The model under review builds one solid part; all positions refer to its coordinate system, in mm. A direction names the side the tool comes from. Round coordinates to 2 decimals unless told otherwise and drop trailing zeros. Order: outer loops, then holes, each group sorted by start corner. A loop starts at its lowest first (then second) coordinate and runs counter-clockwise, first axis right, second up. Notation, with made-up numbers: M 25,-13 L 78,-13 A22 cw 78,-6 Z; hole C 78.25,66.25 d6. An arc over 180 degrees is marked long. Answer as CSV lines item,"result". Start each with the question number.
from build123d import *

# Parameters (mm, degrees)
SKETCH2_W         = 27.0256
SKETCH2_H         = 28.448
MOUNT_BLOCK_DEPTH = 22.2123
MID_HEX_DEPTH     = 20.7645
SKETCH4_R         = 4.233333333
SKETCH4_R_2       = 3.175
SWGLK_M_DEPTH     = 10.287
SKETCH6_R         = 6.35
SKETCH6_R_2       = 3.175
SKETCH7_R         = 2.05105
MOUNT_HOLES_DEPTH = 12.7


with BuildPart() as part:
    # Sketch1 → BASE (revolve)
    with BuildSketch(Plane(origin=(0, 0, 0), x_dir=(0, 0, -1), z_dir=(1, 0, 0)), mode=Mode.PRIVATE) as base_sk:
        Polygon((0, 0), (12.7, 0), (12.7, 22.2123), (14.21765, 22.2123), (14.21765, 42.9768), (9.4234, 42.9768), (9.4234, 51.0667), (26.924, 51.0667), (26.924, 99.1743), (0, 99.1743), align=None)
    revolve(base_sk.sketch.rotate(Axis((0, 0, 0), (0, -1, 0)), 180), axis=Axis((0, 0, 0), (0, -1, 0)))

    # Sketch2 → MOUNT_BLOCK (add)
    with BuildSketch(Plane.XZ):
        Rectangle(SKETCH2_W, SKETCH2_H)
    extrude(amount=-MOUNT_BLOCK_DEPTH)

    # Sketch3 → MID_HEX (add)
    with BuildSketch(Plane.XZ.offset(-22.2123)):
        Polygon((16.417128109, 0), (8.208564055, 14.21765), (-8.208564055, 14.21765), (-16.417128109, 0), (-8.208564055, -14.21765), (8.208564055, -14.21765), align=None)
    extrude(amount=-MID_HEX_DEPTH)

    # Sketch4 → SWGLK_M (add)
    with BuildSketch(Plane.XY.offset(14.224)):
        with Locations((0, 11.10615)):
            Circle(SKETCH4_R)
        with Locations((0, 11.10615)):
            Circle(SKETCH4_R_2, mode=Mode.SUBTRACT)
    swglk_m = extrude(amount=SWGLK_M_DEPTH)

    # SWGLK_M_MRR: SWGLK_M across plane
    add(swglk_m.mirror(Plane.XY))

    # PRESS_QD: sweep along a path in Sketch5
    with BuildLine(Plane(origin=(0, 0, 0), x_dir=(0, 0, -1), z_dir=(1, 0, 0))) as press_qd_path:
        Line((0, 99.1743), (0, 111.76762))
        ThreePointArc((0, 111.76762), (2.789807909, 118.502812091), (9.525, 121.29262))
        Line((9.525, 121.29262), (19.05, 121.29262))
    # Sketch6 → PRESS_QD (sweep)
    with BuildSketch(Plane(origin=(0, 99.1743, 0), x_dir=(1, 0, 0), z_dir=(0, 1, 0))):
        Circle(SKETCH6_R)
        Circle(SKETCH6_R_2, mode=Mode.SUBTRACT)
    sweep(path=press_qd_path.line)

    # Sketch7 → MOUNT_HOLES (cut)
    with BuildSketch(Plane.XZ):
        with Locations(Location((-8.296007071, -9.60755, 0), (0, 0, 270))):
            Circle(SKETCH7_R)
        with Locations(Location((8.296007071, 9.60755, 0), (0, 0, 270))):
            Circle(SKETCH7_R)
    extrude(amount=-MOUNT_HOLES_DEPTH, mode=Mode.SUBTRACT)


solid = part.part
Item 1: Tool access review of faces 5 (the flat face through (12.255, 32.449, -7.208)), 6 (the cylindrical face through (7.51, 6.261, 7.713)), 7 (the cylindrical face through (-0.414, 47.078, -9.414)), 8 (the flat face through (13.513, 11, 0)), 9 (the flat face through (0, 6, 14.224)): name each direction out of +Z, -Z, +X, -X, +Y, -Y from which nothing blocks a thin tool from reaching the whole face with its end or side.
Item 2: The part is to be moulded in two halves that separate along X. For faces 1 (the flat face through (-8, 12.7, -10)), 2 (the flat face through (0, 51.067, -12)), 3 (the cylindrical face through (-1.38, 127.49, -14.35)), 4 (the cylindrical face through (1.47, 8.29, -19.3)), say which applies: +X half, -X half, draft (parallel to the pull), parting line (faces both ways), or undercut.
Item 3: Consider section B-B (y = 83.5). State the section outline as (x, z) points, and give its area (3 significant figures).
Item 4: Consider section C-C (x = -23). State the section outline as (y, z) points, and give its area (3 significant figures).
Item 5: For pin 1 (4 mm diameter, centred on x = -5, z = 17.5, fed in from +Y); pin 2 (13 mm diameter, centred on x = -1.5, y = 37, fed in from -Z); pin 3 (6 mm diameter, centred on y = 71, z = -2.5, fed in from +X), all flat-tipped, find the tip position at first contact; note any pin that passes through.
Item 6: Wall thickness on probe 1 along Y at (x, z) = (0, -13.25); probe 2 along Y at (x, z) = (0, -18.25); probe 3 along Y at (x, z) = (9.5, 8): over which ranges is each line inside the solid? List them lowest first. Write a range as [from, to].
Item 7: Consider section A-A (z = -16.5). State the section outline as (x, y) points (3 decimals), and give its area (3 significant figures).
Item 8: Consider section D-D (y = 47). State the section outline as (x, z) points, and give its area (3 significant figures).
Reported:
1,face 5,"-Z, +X"
1,face 6,"-Y"
1,face 7,"none"
1,face 8,"+Z, -Z, +X, -Y"
1,face 9,"+Z"
2,face 1,"undercut"
2,face 2,"draft"
2,face 3,"parting line"
2,face 4,"undercut"
3,outline,"C 0,0 d53.85"
3,area,"2,280 mm²"
4,outline,"M 51.07,-14 L 99.17,-14 L 99.17,14 L 51.07,14 Z"
4,area,"1,350 mm²"
5,pin 1,"stops at y = 99.17"
5,pin 2,"stops at z = -14.22"
5,pin 3,"stops at x = 26.92"
6,probe 1,"y = [0, 42.98], [51.07, 99.17], [114.94, 118.12], [124.47, 127.64]"
6,probe 2,"y = [6.87, 7.93], [14.28, 15.34], [51.07, 99.17], [114.94, 118.12], [124.47, 127.64]"
6,probe 3,"y = [12.7, 42.98], [51.07, 99.17]"
7,outline,"M -21.276,51.067 L 21.276,51.067 L 21.276,99.174 L -21.276,99.174 Z; C 0,121.293 d12.7; C 0,11.106 d8.467; hole C 0,11.106 d6.35; hole C 0,121.293 d6.35"
7,area,"2,170 mm²"
8,outline,"C 0,0 d18.85"
8,area,"279 mm²"
